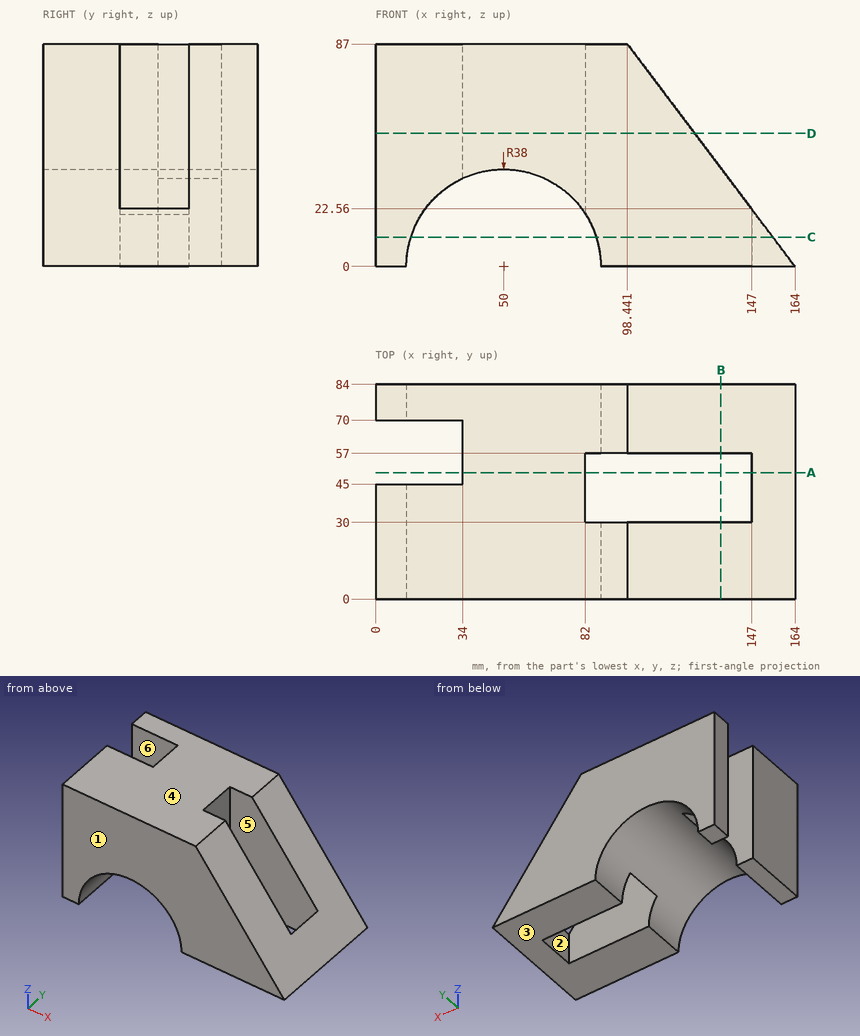
Study the drawing (mm; zero at the part's minimum x, y, z) and answer. A direction names the side the tool comes from. Give positions to 0.01 mm unless a question says otherwise; leave off trailing zeros. Loops run counter-clockwise (first coordinate to the right, second up) from the corner with the lowest first, then second, coordinate; pieces in that order, holes last. Notation, with made-up numbers: M -19,66 L -12,66 A25 cw -12,97 Z; hole C 51,3.5 d7. An arc over 180 degrees is marked long. One line per item, written item: value. Start each with the question number.
1. Find section A-A (y = 49.5). Give the vertices of the cut face in (x, z), and give its area (3 significant figures).
2. Find section D-D (z = 52). Give the vertices of the cut face in (x, y) (1 decimal).
3. Find section C-C (z = 11.5). Give the vertices of the cut face in (x, y), and give its area (3 significant figures).
4. Each of these flat-tipped pins is pushed along its axis until it touches: P1, Ø12, axis at x = 130, z = 60.5, coming from the -Y side; P2, Ø12, axis at y = 26, z = 59.5, coming from the +X side (1 decimal); P3, Ø12.5, axis at y = 58.5, z = 55, coming from the -X side; P4, Ø1.5, axis at y = 17, z = 44.5, coming from the +X side. Where does it stop, or does it pass through?
5. Find the intervals of material crossed by probe 1 along Y at (x, z) = (108.5, 5); probe 2 along Y at (x, z) = (30, 64); probe 3 along X at (y, z) = (38, 21) (1 decimal), in increasing order.
6. Find section B-B (x = 135). Give the vertices of the cut face in (y, z), and give its area (3 significant figures).
7. Which of the six approach directions +Z, -Z, +X, -X, +Y, -Y give full straight-line access (tool end or side, diameter ignored) to the marked faces 4, 5 and 6?
8. Determine the mould class of the marked faces 1, 2 and 3 for opening direction Y: released by +Y, released by -Y, zero draft, split by the parting line, or undercut.
Reported:
1. outline: M 34,34.47 A38 cw 82,20.49 L 82,87 L 34,87 Z; M 147,0 L 164,0 L 147,22.56 Z
1. area: 2,730 mm²
2. outline: M 0,0 L 124.8,0 L 124.8,30 L 82,30 L 82,57 L 124.8,57 L 124.8,84 L 0,84 L 0,70 L 34,70 L 34,45 L 0,45 Z
3. outline: M 0,0 L 13.78,0 L 13.78,45 L 0,45 Z; M 0,70 L 13.78,70 L 13.78,84 L 0,84 Z; M 86.22,0 L 155.33,0 L 155.33,84 L 86.22,84 L 86.22,57 L 147,57 L 147,30 L 86.22,30 Z
3. area: 4,980 mm²
4. P1: passes through
4. P2: stops at x = 123.7
4. P3: stops at x = 34
4. P4: stops at x = 131.03
5. probe 1: y = 0 to 30, 57 to 84
5. probe 2: y = 0 to 45, 70 to 84
5. probe 3: x = 0 to 18.3, 81.7 to 82, 147 to 148.2
6. outline: M 0,0 L 30,0 L 30,38.48 L 0,38.48 Z; M 57,0 L 84,0 L 84,38.48 L 57,38.48 Z
6. area: 2,190 mm²
7. face 4: +Z, +X, -X, +Y, -Y
7. face 5: +Z, -Z
7. face 6: +Z, -Z, -X
8. face 1: released by -Y
8. face 2: undercut
8. face 3: zero draft
